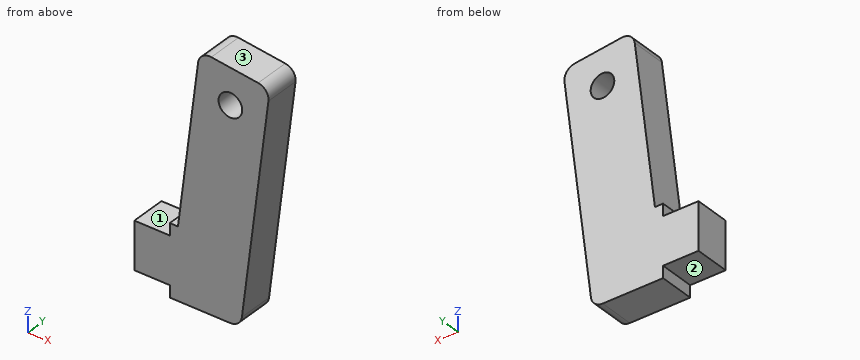
from build123d import *

# Parameters (mm, degrees)
SKETCH2_R           = 1
BOSS_EXTRUDE1_DEPTH = 3
FILLET1_R           = 1


with BuildPart() as part:
    # Sketch2 → Boss-Extrude1 (new body)
    with BuildSketch(Plane(origin=(0, 0, 0), x_dir=(1, 0, 0), z_dir=(0, 1, 0))):
        Polygon((20.748238747, 19.933341623), (14.748238747, 19.933341623), (14.748238747, 18.933341623), (11.748238747, 18.933341623), (11.748238747, 14.933341623), (14.748238747, 14.933341623), (14.748238747, 13.933341623), (15.43988716, 13.933341623), (17.267927311, -0.954850651), (23.22320422, -0.223634591), align=None)
        with Locations(Location((19.879957735, 2.388395834, 0), (0, 0, 270))):
            Circle(SKETCH2_R, mode=Mode.SUBTRACT)
    extrude(amount=BOSS_EXTRUDE1_DEPTH)

    # Fillet1
    fillet1_edges = [part.edges().sort_by_distance(p)[0] for p in [
        (20.748238747, 1.5, -19.933341623),
        (23.22320422, 1.5, 0.223634591),
        (17.267927311, 1.5, 0.954850651),
    ]]
    fillet(fillet1_edges, radius=FILLET1_R)


solid = part.part
Geometry: final body of the model. Coordinates: model frame, mm. Face numbers are marked on the shaded views. A direction names the side the tool comes from. Give positions to 0.01 mm unless a question says otherwise; leave off trailing zeros. Write each loop counter-clockwise with the first axis right and the second up, starting at its lowest first coordinate (ties: lowest second). Pieces come first, ordered by that corner, then holes. Notation, with made-up numbers: (57.5, 86.5) - (76.5, 86.5) arc R9 ccw to (76.5, 92.5) - close; hole circle Ø7 at (40.5, 25.5). An arc over 180 degrees is marked (long way). Return JSON: item names as keys, results as strings. Group by question number.
1) Section A-A on y = 0.8. Return the cut outline in (x, z).
2) Line query: line 1 (Z direction, x = 18, y = 1.35); line 2 (X direction, y = 2.1, z = -3); line 3 (Z direction, x = 14, y = 0.4). Output: solid intervals per line, ascending.
3) First-contact query: P1, Ø0.9, axis at x = 13, y = 2, coming from the +Z side; P2, Ø0.9, axis at x = 13, y = 1.5, coming from the -Z side. Flat tips, straight axial feed; report the tip coordinate or a pass-through.
4) Set-up query: the marked faces 1, 2 and 3. Return all of +Z, -Z, +X, -X, +Y, -Y with unobstructed straight access to the full face (end or side cutting, diameter ignored); none if empty.
5) Section C-C on z = -4.5. Return the cut outline in (x, y).
6) Section B-B on x = 16. Return the cut outline in (y, z).
Filled in:
{
 "1": {"outline": "(11.75, -18.93) - (14.75, -18.93) - (14.75, -19.93) - (19.86, -19.93) arc R1 ccw to (20.86, -19.06) - (23.1, -0.77) arc R1 ccw to (22.23, 0.35) - (18.26, 0.83) arc R1 ccw to (17.15, -0.04) - (15.44, -13.93) - (14.75, -13.93) - (14.75, -14.93) - (11.75, -14.93) - close; hole circle Ø2 at (19.88, -2.39)"},
 "2": {"line 1": "z = -19.93 to 0.83", "line 2": "x = 16.78 to 19.09, 20.67 to 22.83", "line 3": "z = -18.93 to -14.93"},
 "3": {"P1": "stops at z = -14.93", "P2": "stops at z = -18.93"},
 "4": {"face 1": "+Z, -X, +Y, -Y", "face 2": "-Z, -X, +Y, -Y", "face 3": "+Z, +X, +Y, -Y"},
 "5": {"outline": "(16.6, 0) - (22.64, 0) - (22.64, 3) - (16.6, 3) - close"},
 "6": {"outline": "(0, -19.93) - (3, -19.93) - (3, -9.37) - (0, -9.37) - close"}
}
